Part model, mm, in its own coordinate system. Give positions to 0.01 mm unless a question says otherwise; leave off trailing zeros. Order: outer loops, then holes, each group sorted by start corner. A loop starts at its lowest first (then second) coordinate and runs counter-clockwise, first axis right, second up. Notation, with made-up numbers: (68.25, 59.25) - (85.25, 59.25) arc R31 ccw to (85.25, 85.25) - close; hole circle Ø4 at (-6, 21). An arc over 180 degrees is marked (long way). One line per item, written item: value.
```python
from build123d import *

# Parameters (mm, degrees)
F1_DEPTH  = 4
F3_D      = 3.5
F3_DEPTH  = 4
F5_D      = 4.5
F5_DEPTH  = 4
F7_D      = 8
F7_DEPTH  = 4
F9_D      = 8
F9_DEPTH  = 4
F11_D     = 5
F11_DEPTH = 4
F13_D     = 3.5
F13_DEPTH = 4
F15_D     = 3.5
F15_DEPTH = 4
F17_D     = 3.5
F17_DEPTH = 4
F19_D     = 3.5
F19_DEPTH = 4
F21_D     = 3.5
F21_DEPTH = 4
F23_D     = 3.5
F23_DEPTH = 4
F25_D     = 5
F25_DEPTH = 4
F27_D     = 5
F27_DEPTH = 4
F29_D     = 5
F29_DEPTH = 4
F31_D     = 8
F31_DEPTH = 4
F33_D     = 8
F33_DEPTH = 4
F35_D     = 3.5
F35_DEPTH = 4
F37_D     = 3.5
F37_DEPTH = 4


with BuildPart() as f1:
    # F0 (on Top) → F1 (new body)
    with BuildSketch(Plane.XY):
        Polygon((-90, 51.605066), (-90, -39.394934), (-90, -130.394934), (-40, -130.394934), (-40, -198.394934), (-90, -198.394934), (-90, -242.394934), (0, -267.623484), (90, -242.394934), (90, -198.394934), (40, -198.394934), (40, -130.394934), (90, -130.394934), (90, -39.394934), (90, 51.605066), (40, 51.605066), (40, 121.605066), (90, 121.605066), (90, 155.605066), (0, 193.605066), (-90, 155.605066), (-90, 121.605066), (-40, 121.605066), (-40, 51.605066), align=None)
    extrude(amount=F1_DEPTH)

    # F3
    with Locations(Plane.XY.offset(4)):
        with Locations((0, 187.605066)):
            Hole(F3_D / 2, depth=F3_DEPTH)

    # F5
    with Locations(Plane.XY.offset(4)):
        with Locations((0, 105.605066)):
            Hole(F5_D / 2, depth=F5_DEPTH)

    # F7
    with Locations(Plane.XY.offset(4)):
        with Locations((-20, 65.605066)):
            Hole(F7_D / 2, depth=F7_DEPTH)

    # F9
    with Locations(Plane.XY.offset(4)):
        with Locations((20, 65.605066)):
            Hole(F9_D / 2, depth=F9_DEPTH)

    # F11
    with Locations(Plane.XY.offset(4)):
        with Locations((28, 47.605066)):
            Hole(F11_D / 2, depth=F11_DEPTH)

    # F13
    with Locations(Plane.XY.offset(4)):
        with Locations((45, 19.605066)):
            Hole(F13_D / 2, depth=F13_DEPTH)

    # F15
    with Locations(Plane.XY.offset(4)):
        with Locations((45, -32.394934)):
            Hole(F15_D / 2, depth=F15_DEPTH)

    # F17
    with Locations(Plane.XY.offset(4)):
        with Locations((45, -90.394934)):
            Hole(F17_D / 2, depth=F17_DEPTH)

    # F19
    with Locations(Plane.XY.offset(4)):
        with Locations((-44, 19.605066)):
            Hole(F19_D / 2, depth=F19_DEPTH)

    # F21
    with Locations(Plane.XY.offset(4)):
        with Locations((-44, -32.394934)):
            Hole(F21_D / 2, depth=F21_DEPTH)

    # F23
    with Locations(Plane.XY.offset(4)):
        with Locations((-44, -90.394934)):
            Hole(F23_D / 2, depth=F23_DEPTH)

    # F25
    with Locations(Plane.XY.offset(4)):
        with Locations((-14, -5.904332)):
            Hole(F25_D / 2, depth=F25_DEPTH)

    # F27
    with Locations(Plane.XY.offset(4)):
        with Locations((-14, -65.016279)):
            Hole(F27_D / 2, depth=F27_DEPTH)

    # F29
    with Locations(Plane.XY.offset(4)):
        with Locations((28, -127.623484)):
            Hole(F29_D / 2, depth=F29_DEPTH)

    # F31
    with Locations(Plane.XY.offset(4)):
        with Locations((20, -141.623484)):
            Hole(F31_D / 2, depth=F31_DEPTH)

    # F33
    with Locations(Plane.XY.offset(4)):
        with Locations((-20, -141.623484)):
            Hole(F33_D / 2, depth=F33_DEPTH)

    # F35
    with Locations(Plane.XY.offset(4)):
        with Locations((-17.5, -157.623484)):
            Hole(F35_D / 2, depth=F35_DEPTH)

    # F37
    with Locations(Plane.XY.offset(4)):
        with Locations((17.5, -157.623484)):
            Hole(F37_D / 2, depth=F37_DEPTH)


solid = f1.part
```
1) Slice it at A-A on x = 70. Write the cut outline in (y, z).
Answer:
outline: (-248, 0) - (-198.39, 0) - (-198.39, 4) - (-248, 4) - close; (-130.39, 0) - (51.61, 0) - (51.61, 4) - (-130.39, 4) - close; (121.61, 0) - (164.05, 0) - (164.05, 4) - (121.61, 4) - close
2) Wall check: line 1 along Y through (x, z) = (54, 2.9); line 2 along Y through (x, z) = (-82, 2.8); line 3 along X through (y, z) = (-139, 3.45). Give the ranges that are in metal, low to high. Write a range as [from, to].
Answer:
line 1: y = [-252.49, -198.39], [-130.39, 51.61], [121.61, 170.81]
line 2: y = [-244.64, -198.39], [-130.39, 51.61], [121.61, 158.98]
line 3: x = [-40, -23.02], [-16.98, 16.98], [23.02, 40]
3) Slice it at B-B on z = 3.4. Count the separate pieces of the cut face and the enclosed holes in it, then the cut area to 3 significant figures.
Answer:
separate pieces: 1
enclosed holes: 18
area: 63,100 mm2
4) Drop flat-ended pins along their axis: P1, Ø1, axis at x = -35.5, z = 0.5, coming from the +Y side; P2, Ø1.2, axis at y = -164.5, z = 3, coming from the -X side; P3, Ø1.2, axis at x = 63, z = 1, coming from the -Y side. Give the stop position or say it passes through.
Answer:
P1: stops at y = 178.83
P2: stops at x = -40
P3: stops at y = -250.13
5) Two-plate mould, pull along X, no slides. Class faces 1 (the face through (-45.63, -254.833, 1.972)), 2 (the face through (-19.13, 61.7, 1.97)), 3 (the face through (-1, -34, 0)): pulls with the +X half, pulls with the -X half, needs draft (parallel to the pull), parting line crosses it, or undercut.
Answer:
face 1: pulls with the -X half
face 2: undercut
face 3: needs draft
